from build123d import *

# Parameters (mm, degrees)
SKETCH2_W           = 57.15
SKETCH2_H           = 6.35
SKETCH3_R           = 19.05
BOSS_EXTRUDE1_DEPTH = 50.8
SKETCH4_R           = 6.35
CUT_EXTRUDE1_DEPTH  = 81.026


with BuildPart() as part:
    # Sketch2 → Revolve1 (revolve)
    with BuildSketch(Plane.XY, mode=Mode.PRIVATE) as revolve1_sk:
        with Locations((28.575, -3.175)):
            Rectangle(SKETCH2_W, SKETCH2_H)
    revolve(revolve1_sk.sketch.rotate(Axis((0, 0, 0), (0, -1, 0)), 90), axis=Axis((0, 0, 0), (0, -1, 0)))

    # Sketch3 → Boss-Extrude1 (add)
    with BuildSketch(Plane(origin=(0, 0, 0), x_dir=(1, 0, 0), z_dir=(0, 1, 0))):
        with Locations(Location((0, 0, 0), (0, 0, 270))):
            Circle(SKETCH3_R)
    extrude(amount=BOSS_EXTRUDE1_DEPTH)

    # Sketch4 → Cut-Extrude1 (cut)
    with BuildSketch(Plane(origin=(0, 50.8, 0), x_dir=(1, 0, 0), z_dir=(0, 1, 0))):
        with Locations(Location((0, 0, 0), (0, 0, 270))):
            Circle(SKETCH4_R)
    extrude(amount=-CUT_EXTRUDE1_DEPTH, mode=Mode.SUBTRACT)


solid = part.part
Check sheet for the modelled part. Datum: model origin and axes. Units: mm. A direction names the side the tool comes from. Round coordinates to 2 decimals unless told otherwise and drop trailing zeros. Write each loop counter-clockwise with the first axis right and the second up, starting at its lowest first coordinate (ties: lowest second). Pieces come first, ordered by that corner, then holes. Notation, with made-up numbers: (7.5, 67.25) -> (34.5, 67.25) arc R23 cw to (34.5, 86.25) -> close; hole circle Ø2 at (23.25, -36). An arc over 180 degrees is marked (long way). Answer as CSV lines item,"result". Start each with the question number.
1) Section check D-D on z = -36. Enter the section's corners in (x, y).
2) Release check for a two-part mould opening along X. For faces 1 (the cylindrical face through (-2.513, -3.131, -57.095)), 2 (the flat face through (12, -6.35, 1)), 3 (the cylindrical face through (-3.86, 22.63, -5.04)) record: pulls with the +X half, pulls with the -X half, needs draft (parallel to the pull), parting line crosses it, or undercut.
3) Material ranges on line 1 (X direction, y = 34.5, z = 0); line 2 (Y direction, x = 51, z = 25); line 3 (X direction, y = 38, z = 1.5), recorded low to high. Write a range as from..to.
4) Tool access check on faces 4 (the cylindrical face through (-11.59, 25.04, -15.12)), 5 (the flat face through (5, 50.8, -5)). Record the directions out of +Z, -Z, +X, -X, +Y, -Y that give a thin tool (end or side, any length) a straight path to the whole face; none if there is none.
5) Section check A-A on z = 0. Enter the section's corners in (x, y).
6) Section check C-C on y = 43. Enter the section's corners in (x, z).
7) Go/stop test with flat-tipped pins: P1, Ø3, axis at x = 9, y = 42.5, coming from the -Z side; P2, Ø16.5, axis at x = 0, z = 0, coming from the +Y side; P3, Ø1, axis at x = 30, z = 28.5, coming from the +Y side; P4, Ø10, axis at x = 18, y = 39.5, coming from the -Z side. Record where each tip stops, or that it passes through.
8) Section check B-B on x = 0. Enter the section's corners in (y, z), and give its area (3 significant figures).
Found:
1,outline,"(-44.39, -6.35) -> (44.39, -6.35) -> (44.39, 0) -> (-44.39, 0) -> close"
2,face 1,"parting line crosses it"
2,face 2,"needs draft"
2,face 3,"undercut"
3,line 1,"x = -19.05..-6.35, 6.35..19.05"
3,line 2,"y = -6.35..0"
3,line 3,"x = -18.99..-6.17, 6.17..18.99"
4,face 4,"+Y"
4,face 5,"+Z, -Z, +X, -X, +Y"
5,outline,"(-57.15, -6.35) -> (-6.35, -6.35) -> (-6.35, 50.8) -> (-19.05, 50.8) -> (-19.05, 0) -> (-57.15, 0) -> close; (6.35, -6.35) -> (57.15, -6.35) -> (57.15, 0) -> (19.05, 0) -> (19.05, 50.8) -> (6.35, 50.8) -> close"
6,outline,"circle Ø38.1 at (0, 0); hole circle Ø12.7 at (0, 0)"
7,P1,"stops at z = -17.51"
7,P2,"stops at y = 50.8"
7,P3,"stops at y = 0"
7,P4,"stops at z = -13.92"
8,outline,"(-6.35, -57.15) -> (0, -57.15) -> (0, -19.05) -> (50.8, -19.05) -> (50.8, -6.35) -> (-6.35, -6.35) -> close; (-6.35, 6.35) -> (50.8, 6.35) -> (50.8, 19.05) -> (0, 19.05) -> (0, 57.15) -> (-6.35, 57.15) -> close"
8,area,"1,940 mm^2"
